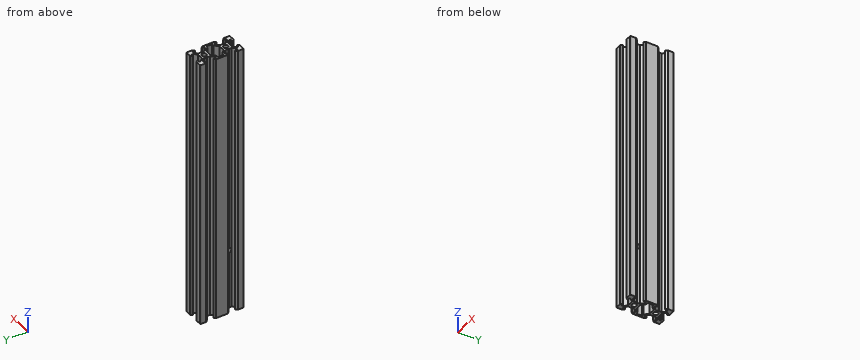
```python
from build123d import *

# Parameters (mm, degrees)
ESBO_O1_R                = 2.1
RESSALTO_EXTRUS_O1_DEPTH = 250
CORTE_EXTRUS_O1_REACH    = 253.595
ESBO_O2_R                = 2.5


with BuildPart() as part:
    # Esboço1 → Ressalto-extrusão1 (new body)
    with BuildSketch(Plane.XY):
        with BuildLine():
            Line((3.9, 9.79), (3.69, 10))
            Line((3.69, 10), (3.9, 10.21))
            Line((3.9, 10.21), (3.9, 12.839339828))
            Line((3.9, 12.839339828), (6.560660172, 15.5))
            Line((6.560660172, 15.5), (8.2, 15.5))
            Line((8.2, 15.5), (8.2, 13.125))
            Line((8.2, 13.125), (8.545, 13.125))
            Line((8.545, 13.125), (10, 14.58))
            Line((10, 14.58), (10, 19.5))
            ThreePointArc((10, 19.5), (9.853553391, 19.853553391), (9.5, 20))
            Line((9.5, 20), (4.58, 20))
            Line((4.58, 20), (3.125, 18.545))
            Line((3.125, 18.545), (3.125, 18.2))
            Line((3.125, 18.2), (5.5, 18.2))
            Line((5.5, 18.2), (5.5, 16.560660172))
            Line((5.5, 16.560660172), (2.839339828, 13.9))
            Line((2.839339828, 13.9), (0.21, 13.9))
            Line((0.21, 13.9), (0, 13.69))
            Line((0, 13.69), (-0.21, 13.9))
            Line((-0.21, 13.9), (-2.839339828, 13.9))
            Line((-2.839339828, 13.9), (-5.5, 16.560660172))
            Line((-5.5, 16.560660172), (-5.5, 18.2))
            Line((-5.5, 18.2), (-3.125, 18.2))
            Line((-3.125, 18.2), (-3.125, 18.545))
            Line((-3.125, 18.545), (-4.58, 20))
            Line((-4.58, 20), (-9.5, 20))
            ThreePointArc((-9.5, 20), (-9.853553391, 19.853553391), (-10, 19.5))
            Line((-10, 19.5), (-10, 14.58))
            Line((-10, 14.58), (-8.545, 13.125))
            Line((-8.545, 13.125), (-8.2, 13.125))
            Line((-8.2, 13.125), (-8.2, 15.5))
            Line((-8.2, 15.5), (-6.560660172, 15.5))
            Line((-6.560660172, 15.5), (-3.9, 12.839339828))
            Line((-3.9, 12.839339828), (-3.9, 10.21))
            Line((-3.9, 10.21), (-3.69, 10))
            Line((-3.69, 10), (-3.9, 9.79))
            Line((-3.9, 9.79), (-3.9, 7.160660172))
            Line((-3.9, 7.160660172), (-6.560660172, 4.5))
            Line((-6.560660172, 4.5), (-8.2, 4.5))
            Line((-8.2, 4.5), (-8.2, 6.875))
            Line((-8.2, 6.875), (-8.545, 6.875))
            Line((-8.545, 6.875), (-10, 5.42))
            Line((-10, 5.42), (-10, -5.42))
            Line((-10, -5.42), (-8.545, -6.875))
            Line((-8.545, -6.875), (-8.2, -6.875))
            Line((-8.2, -6.875), (-8.2, -4.5))
            Line((-8.2, -4.5), (-6.560660172, -4.5))
            Line((-6.560660172, -4.5), (-3.9, -7.160660172))
            Line((-3.9, -7.160660172), (-3.9, -9.79))
            Line((-3.9, -9.79), (-3.69, -10))
            Line((-3.69, -10), (-3.9, -10.21))
            Line((-3.9, -10.21), (-3.9, -12.839339828))
            Line((-3.9, -12.839339828), (-6.560660172, -15.5))
            Line((-6.560660172, -15.5), (-8.2, -15.5))
            Line((-8.2, -15.5), (-8.2, -13.125))
            Line((-8.2, -13.125), (-8.545, -13.125))
            Line((-8.545, -13.125), (-10, -14.58))
            Line((-10, -14.58), (-10, -19.5))
            ThreePointArc((-10, -19.5), (-9.853553391, -19.853553391), (-9.5, -20))
            Line((-9.5, -20), (-4.58, -20))
            Line((-4.58, -20), (-3.125, -18.545))
            Line((-3.125, -18.545), (-3.125, -18.2))
            Line((-3.125, -18.2), (-5.5, -18.2))
            Line((-5.5, -18.2), (-5.5, -16.560660172))
            Line((-5.5, -16.560660172), (-2.839339828, -13.9))
            Line((-2.839339828, -13.9), (-0.21, -13.9))
            Line((-0.21, -13.9), (0, -13.69))
            Line((0, -13.69), (0.21, -13.9))
            Line((0.21, -13.9), (2.839339828, -13.9))
            Line((2.839339828, -13.9), (5.5, -16.560660172))
            Line((5.5, -16.560660172), (5.5, -18.2))
            Line((5.5, -18.2), (3.125, -18.2))
            Line((3.125, -18.2), (3.125, -18.545))
            Line((3.125, -18.545), (4.58, -20))
            Line((4.58, -20), (9.5, -20))
            ThreePointArc((9.5, -20), (9.853553391, -19.853553391), (10, -19.5))
            Line((10, -19.5), (10, -14.58))
            Line((10, -14.58), (8.545, -13.125))
            Line((8.545, -13.125), (8.2, -13.125))
            Line((8.2, -13.125), (8.2, -15.5))
            Line((8.2, -15.5), (6.560660172, -15.5))
            Line((6.560660172, -15.5), (3.9, -12.839339828))
            Line((3.9, -12.839339828), (3.9, -10.21))
            Line((3.9, -10.21), (3.69, -10))
            Line((3.69, -10), (3.9, -9.79))
            Line((3.9, -9.79), (3.9, -7.160660172))
            Line((3.9, -7.160660172), (6.560660172, -4.5))
            Line((6.560660172, -4.5), (8.2, -4.5))
            Line((8.2, -4.5), (8.2, -6.875))
            Line((8.2, -6.875), (8.545, -6.875))
            Line((8.545, -6.875), (10, -5.42))
            Line((10, -5.42), (10, 5.42))
            Line((10, 5.42), (8.545, 6.875))
            Line((8.545, 6.875), (8.2, 6.875))
            Line((8.2, 6.875), (8.2, 4.5))
            Line((8.2, 4.5), (6.560660172, 4.5))
            Line((6.560660172, 4.5), (3.9, 7.160660172))
            Line((3.9, 7.160660172), (3.9, 9.79))
        make_face()
        with Locations((0, -10)):
            Circle(ESBO_O1_R, mode=Mode.SUBTRACT)
        with Locations((0, 10)):
            Circle(ESBO_O1_R, mode=Mode.SUBTRACT)
        Polygon((8.2, -2.7), (8.2, 2.7), (6.239339828, 2.7), (2.839339828, 6.1), (-2.839339828, 6.1), (-6.239339828, 2.7), (-8.2, 2.7), (-8.2, -2.7), (-6.239339828, -2.7), (-2.839339828, -6.1), (2.839339828, -6.1), (6.239339828, -2.7), align=None, mode=Mode.SUBTRACT)
    extrude(amount=RESSALTO_EXTRUS_O1_DEPTH)

    # Corte-extrusão1: up to this face of the body (flat: up to its plane)
    corte_extrus_o1_end = Plane(part.part.faces().sort_by_distance((-10, 0, 125))[0])
    # Esboço2 → Corte-extrusão1 (cut, up to the picked face)
    with BuildSketch(Plane(origin=(10, 0, 0), x_dir=(0, 0, -1), z_dir=(1, 0, 0)), mode=Mode.PRIVATE) as corte_extrus_o1_sk1:
        with Locations((-55, -10)):
            Circle(ESBO_O2_R)
    corte_extrus_o1_tool1 = split(extrude(corte_extrus_o1_sk1.sketch, amount=-CORTE_EXTRUS_O1_REACH, mode=Mode.PRIVATE), bisect_by=corte_extrus_o1_end, keep=Keep.BOTH, mode=Mode.PRIVATE)
    add(corte_extrus_o1_tool1.solids().sort_by(Axis((10, -10, 55), (-1, 0, 0)))[0], mode=Mode.SUBTRACT)


solid = part.part
```
Part model, mm, in its own coordinate system. Round coordinates to 2 decimals unless told otherwise and drop trailing zeros. Use one line per item in the form item = value. Start each with the question number.
Item 1: Drop flat-ended pins along their axis: pin 1 Ø2.5 at (x, z) = (4.5, 146) entering from -Y; pin 2 Ø1 at (y, z) = (12.5, 178) entering from +X; pin 3 Ø0.8 at (y, z) = (8, 171) entering from -X; pin 4 Ø2 at (x, z) = (-1, 69.5) entering from +Y. Give the stop position or say it passes through.
Item 2: Band-saw the part on A-A (z = 28.5). Give the number of separate pieces and of enclosed holes in the cut face, plus the area to 3 significant figures.
Item 3: Drill centre lines: line 1 along Y through (x, z) = (-6.75, 94); line 2 along Y through (x, z) = (0, 154); line 3 along X through (y, z) = (5, 31). Where is each one in solid material? Low to high.
Data:
q1.pin_1 = -20
q1.pin_2 = 4.06
q1.pin_3 = -3.9
q1.pin_4 = 13.9
q2.separate_pieces = 1
q2.enclosed_holes = 3
q2.area = 300 mm^2
q3.line_1 = -20 to -15.5, -4.5 to -2.7, 2.7 to 4.5, 15.5 to 20
q3.line_2 = -13.69 to -12.1, -7.9 to -6.1, 6.1 to 7.9, 12.1 to 13.69
q3.line_3 = -10 to -8.2, -6.06 to -3.94, 3.94 to 6.06, 8.2 to 10
